Input: part model. Units: mm. Frame: model coordinates. Face numbers are marked on the shaded views. A direction names the side the tool comes from. Give positions to 0.01 mm unless a question says otherwise; leave off trailing zeros. Order: outer loops, then holes, each group sorted by start corner. A loop starts at its lowest first (then second) coordinate and runs counter-clockwise, first axis right, second up. Notation, with made-up numbers: M -10.5,-15.5 L 48.5,-15.5 A12 cw 48.5,5.5 Z; hole C 63.5,21 d3. An arc over 180 degrees is marked long. Use a Markdown table: item, result.
from build123d import *

# Parameters (mm, degrees)
SKETCH_1_R       = 18.5
EXTRUDE_3_DEPTH  = 23
SKETCH_3_R       = 16.5
EXTRUDE_4_DEPTH  = 23
SKETCH_4_R       = 6
EXTRUDE_5_DEPTH  = 6
SKETCH_6_R       = 3
EXTRUDE_6_DEPTH  = 12
SKETCH_7_R       = 2
EXTRUDE_7_DEPTH  = 2
SKETCH_8_W       = 3
SKETCH_8_H       = 1
EXTRUDE_8_DEPTH  = 7
SKETCH_9_R       = 16.5
EXTRUDE_9_DEPTH  = 2
SKETCH_10_W      = 4.5
SKETCH_10_H      = 12
EXTRUDE_10_DEPTH = 5
FILLET_1_R       = 1
SKETCH_11_R      = 8
EXTRUDE_11_DEPTH = 4


with BuildPart() as part:
    # 草图1 → 凸台-拉伸3 (new body)
    with BuildSketch(Plane.XY):
        Circle(SKETCH_1_R)
    extrude(amount=EXTRUDE_3_DEPTH)

    # 草图3 → 凸台-拉伸4 (add)
    with BuildSketch(Plane.XY.offset(23)):
        Circle(SKETCH_3_R)
    extrude(amount=EXTRUDE_4_DEPTH)

    # 草图4 → 凸台-拉伸5 (add)
    with BuildSketch(Plane(origin=(0, 0, 0), x_dir=(-1, 0, 0), z_dir=(0, 0, -1))):
        with Locations(Location((0, 7, 0), (0, 0, 180))):
            Circle(SKETCH_4_R)
    extrude(amount=EXTRUDE_5_DEPTH)

    # 草图6 → 凸台-拉伸6 (add)
    with BuildSketch(Plane(origin=(0, 0, -6), x_dir=(-1, 0, 0), z_dir=(0, 0, -1))):
        with Locations((0, 7)):
            Circle(SKETCH_6_R)
    extrude(amount=EXTRUDE_6_DEPTH)

    # 草图7 → 凸台-拉伸7 (add)
    with BuildSketch(Plane.XY.offset(46)):
        Circle(SKETCH_7_R)
    extrude(amount=EXTRUDE_7_DEPTH)

    # 草图8 → 凸台-拉伸8 (add)
    with BuildSketch(Plane.XY.offset(46)):
        with Locations((0, -12)):
            Rectangle(SKETCH_8_W, SKETCH_8_H)
        with Locations((0.066509227, 12)):
            Rectangle(SKETCH_8_W, SKETCH_8_H)
    extrude(amount=EXTRUDE_8_DEPTH)

    # 草图9 → 凸台-拉伸9 (add)
    with BuildSketch(Plane.XY.offset(48)):
        Circle(SKETCH_9_R)
    extrude(amount=EXTRUDE_9_DEPTH)

    # 草图10 → 凸台-拉伸10 (add)
    with BuildSketch(Plane.XY.offset(50)):
        with Locations((15, 0)):
            Rectangle(SKETCH_10_W, SKETCH_10_H)
    extrude(amount=EXTRUDE_10_DEPTH)

    # 圆角1
    fillet_1_edges = [part.edges().sort_by_distance(p)[0] for p in [
        (1.566509227, 12, 53),
        (-1.433490773, 12, 53),
        (1.5, -12, 53),
        (-1.5, -12, 53),
    ]]
    fillet(fillet_1_edges, radius=FILLET_1_R)

    # 草图11 → 凸台-拉伸11 (add)
    with BuildSketch(Plane.XY.offset(50)):
        Circle(SKETCH_11_R)
    extrude(amount=EXTRUDE_11_DEPTH)


solid = part.part
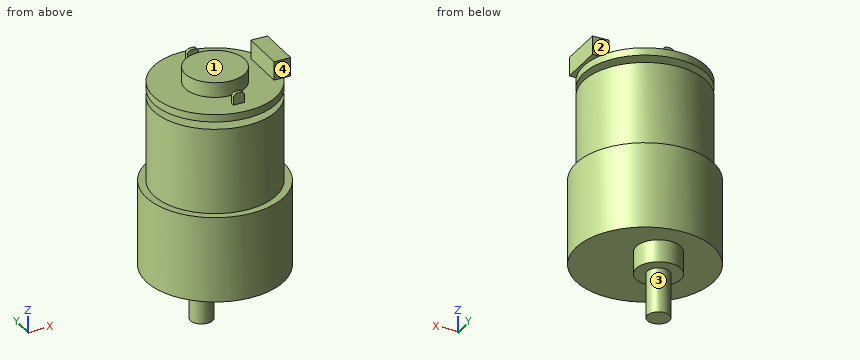
1) Cut plane C-C on z = -11. Return loops of the section in (x, y), and give its area (3 significant figures).
Response values:
| item | result |
|---|---|
| outline | C 0,7 d6 |
| area | 28.3 mm² |
2) Cut plane B-B on x = -10.5. Return loops of the section in (y, z), and give its area (3 significant figures).
Response values:
| item | result |
|---|---|
| outline | M -15.23,0 L 15.23,0 L 15.23,23 L 12.73,23 L 12.73,46 L -12.73,46 L -12.73,23 L -15.23,23 Z; M -12.73,48 L 12.73,48 L 12.73,50 L -12.73,50 Z |
| area | 1,340 mm² |
3) First-contact query: pin 1 Ø0.5 at (y, z) = (-12, 51.5) entering from -X; pin 2 Ø9.5 at (x, y) = (-1, 6) entering from +Z; pin 3 Ø2.5 at (x, z) = (-0.5, 51.5) entering from -Y. Flat tips, straight axial feed; report the tip coordinate or a pass-through.
Response values:
| item | result |
|---|---|
| pin 1 | stops at x = -1.5 |
| pin 2 | stops at z = 54 |
| pin 3 | stops at y = -12.5 |
4) Reachability of the marked faces 1, 2, 3 and 4 from +Z, -Z, +X, -X, +Y, -Y: full face, straight path, thin tool, end or side. Return the list, or none.
Response values:
| item | result |
|---|---|
| face 1 | +Z, -X, +Y, -Y |
| face 2 | +Z, +X, +Y |
| face 3 | -Z |
| face 4 | +Z, +X, -Y |
5) Cut plane D-D on z = 10.5. Return loops of the section in (x, y).
Response values:
| item | result |
|---|---|
| outline | C 0,0 d37 |
6) Cut plane A-A on y = 9. Return loops of the section in (x, z), and give its area (3 significant figures).
Response values:
| item | result |
|---|---|
| outline | M -16.16,0 L -5.66,0 L -5.66,-6 L -2.24,-6 L -2.24,-18 L 2.24,-18 L 2.24,-6 L 5.66,-6 L 5.66,0 L 16.16,0 L 16.16,23 L 13.83,23 L 13.83,46 L -13.83,46 L -13.83,23 L -16.16,23 Z; M -13.83,48 L 13.83,48 L 13.83,50 L -13.83,50 Z |
| area | 1,560 mm² |
7) Material intervals for line 1 (Z direction, x = -16, y = -0.5); line 2 (Z direction, x = -3, y = 2.5); line 3 (X direction, y = 13, z = 29), sorted ascending. Write a range as from..to.
Response values:
| item | result |
|---|---|
| line 1 | z = 0..46, 48..50 |
| line 2 | z = -6..46, 48..54 |
| line 3 | x = -10.16..10.16 |
